Here's the drawing with two shaded views (mm, measured from the low corner). I have some questions. Coordinates: 2 decimals unless noted, no trailing zeros. Loops run counter-clockwise (first coordinate to the right, second up) from the corner with the lowest first, then second, coordinate; pieces in that order, holes last. Notation, with made-up numbers: (40, -27) -> (92, -27) arc R26 ccw to (92, 12) -> close; hole circle Ø7 at (11.25, 10.25). An arc over 180 degrees is marked (long way). Answer as a JSON object with one key per item and string values. Group by question number.
Q1. I want a section at C-C on x = 42. Write out the boundary of the cut face in (y, z) (3 decimals).
Q2. I want a section at B-B on z = 2. Write out the boundary of the cut face in (x, y), then the cut area to 3 significant figures.
Q3. I'm going to push flat-ended pins straight in: pin 1 (4 mm diameter, centred on x = 29.5, z = 17, fed in from +Y); pin 2 (10 mm diameter, centred on x = 35, z = 3, fed in from +Y); pin 3 (1.5 mm diameter, centred on x = 48.5, y = 10.5, fed in from +Z). Where does each tip first touch, or does it pass through?
Q4. I want a section at A-A on y = 5.75. Write out the boundary of the cut face in (x, z), then the cut area to 3 significant figures.
Q5. I need wall thicknesses on line 1 (Z direction, x = 62, y = 9.75); line 2 (Y direction, x = 81, z = 9); line 3 (Z direction, x = 68, y = 15.25). Which ranges of each line are inside material? Lowest first, please.
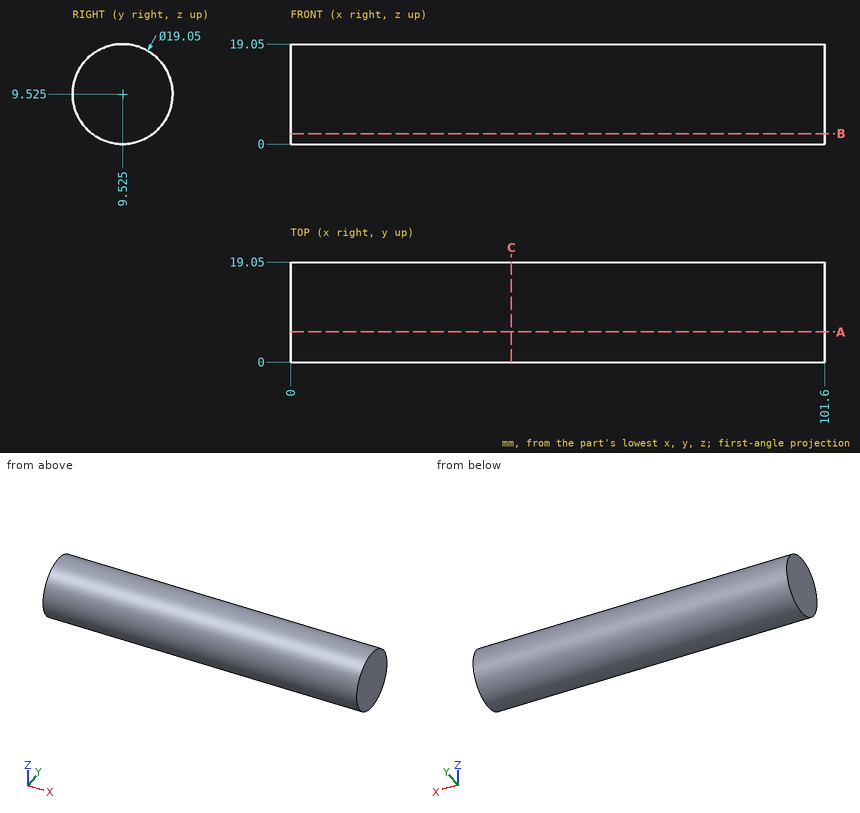
Result set:
{
 "1": {"outline": "circle Ø19.05 at (9.525, 9.525)"},
 "2": {"outline": "(0, 3.69) -> (101.6, 3.69) -> (101.6, 15.36) -> (0, 15.36) -> close", "area": "1,190 mm²"},
 "3": {"pin 1": "stops at y = 17.32", "pin 2": "stops at y = 18.93", "pin 3": "stops at z = 19.05"},
 "4": {"outline": "(0, 0.78) -> (101.6, 0.78) -> (101.6, 18.27) -> (0, 18.27) -> close", "area": "1,780 mm²"},
 "5": {"line 1": "z = 0 to 19.05", "line 2": "y = 0.01 to 19.04", "line 3": "z = 1.91 to 17.14"}
}
